Verification items for this drawing (mm, ordinates from the low corner). A direction names the side the tool comes from. Coordinates: 2 decimals unless noted, no trailing zeros. Loops run counter-clockwise (first coordinate to the right, second up) from the corner with the lowest first, then second, coordinate; pieces in that order, holes last. Notation, with made-up numbers: (20.5, 15.5) - (59.5, 15.5) arc R19 cw to (59.5, 52.5) - close; hole circle Ø5 at (15.5, 27). An arc over 180 degrees is marked (long way). One line per item, written item: value. Start each with the question number.
(1) Draft check along X on the marked faces 3, 4, 5 and 6. Enter one of: +X half, -X half, draft (parallel to the pull), parting line (faces both ways), or undercut.
(2) Gauge pin test, flat ends, axial feed: P1, Ø3.5, axis at y = 6, z = 12, coming from the -X side; P2, Ø0.9, axis at x = 3, z = 22.5, coming from the -Y side; P3, Ø1.5, axis at x = 2.5, z = 12.5, coming from the +Y side; P4, Ø3, axis at x = 23, y = 22, coming from the +Z side. Record the tip position at first contact, or that the pin passes through.
(3) Thickness scan on probe 1 along X at (y, z) = (12.5, 24.5); probe 2 along X at (y, z) = (8.5, 6.5); probe 3 along Z at (x, y) = (22, 23.5). Record the ranges inside material, lowest first. Write a range as [from, to].
(4) Section check A-A (z = 37). Record the boundary of the cut face in (x, y).
(5) Section check B-B (y = 6). Record the boundary of the cut face in (x, z).
(6) Section check D-D (x = 20). Record the boundary of the cut face in (y, z).
(7) Section check C-C (x = 45). Record the boundary of the cut face in (y, z), plus the area to 3 significant figures.
(8) Set-up check for the marked faces 1 and 2: record each of +Z, -Z, +X, -X, +Y, -Y from which the full face is reachable in a straight line by a thin tool's end or side.
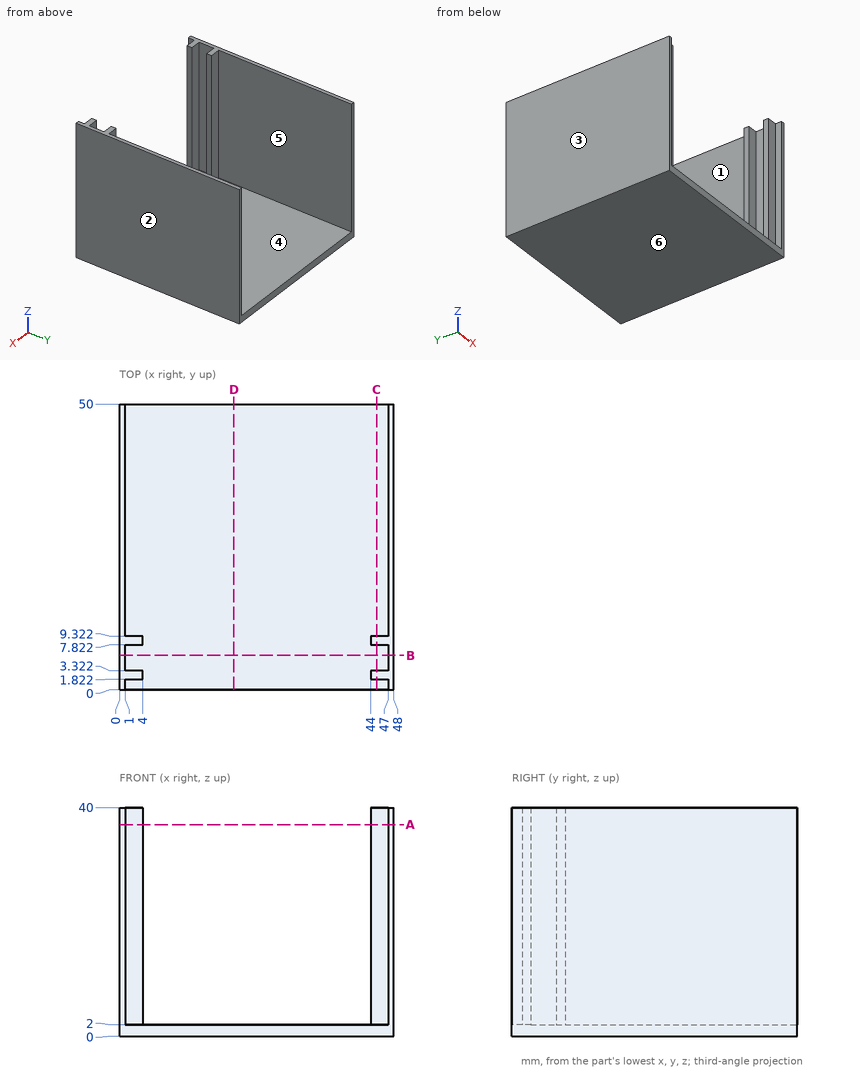
Responses:
1. face 3: -X half
1. face 4: undercut
1. face 5: undercut
1. face 6: draft
2. P1: stops at x = 0
2. P2: stops at y = 1.82
2. P3: stops at y = 9.32
2. P4: stops at z = 2
3. probe 1: x = [0, 1], [47, 48]
3. probe 2: x = [0, 4], [44, 48]
3. probe 3: z = [0, 2]
4. outline: (0, 0) - (1, 0) - (1, 1.82) - (4, 1.82) - (4, 3.32) - (1, 3.32) - (1, 7.82) - (4, 7.82) - (4, 9.32) - (1, 9.32) - (1, 50) - (0, 50) - close; (44, 1.82) - (47, 1.82) - (47, 0) - (48, 0) - (48, 50) - (47, 50) - (47, 9.32) - (44, 9.32) - (44, 7.82) - (47, 7.82) - (47, 3.32) - (44, 3.32) - close
5. outline: (0, 0) - (48, 0) - (48, 40) - (47, 40) - (47, 2) - (1, 2) - (1, 40) - (0, 40) - close
6. outline: (0, 0) - (50, 0) - (50, 2) - (0, 2) - close
7. outline: (0, 0) - (50, 0) - (50, 2) - (9.32, 2) - (9.32, 40) - (7.82, 40) - (7.82, 2) - (3.32, 2) - (3.32, 40) - (1.82, 40) - (1.82, 2) - (0, 2) - close
7. area: 214 mm²
8. face 1: +Z, +Y
8. face 2: +Z, -Z, +X, +Y, -Y
